Verification items for this drawing (mm, ordinates from the low corner). Coordinates: 2 decimals unless noted, no trailing zeros. Loops run counter-clockwise (first coordinate to the right, second up) from the corner with the lowest first, then second, coordinate; pieces in that order, holes last. Notation, with made-up numbers: (-35, 58) -> (24, 58) arc R13 ccw to (24, 75) -> close; hole circle Ø7 at (48, 17.25). An arc over 180 degrees is marked (long way). Write item = value, one per line.
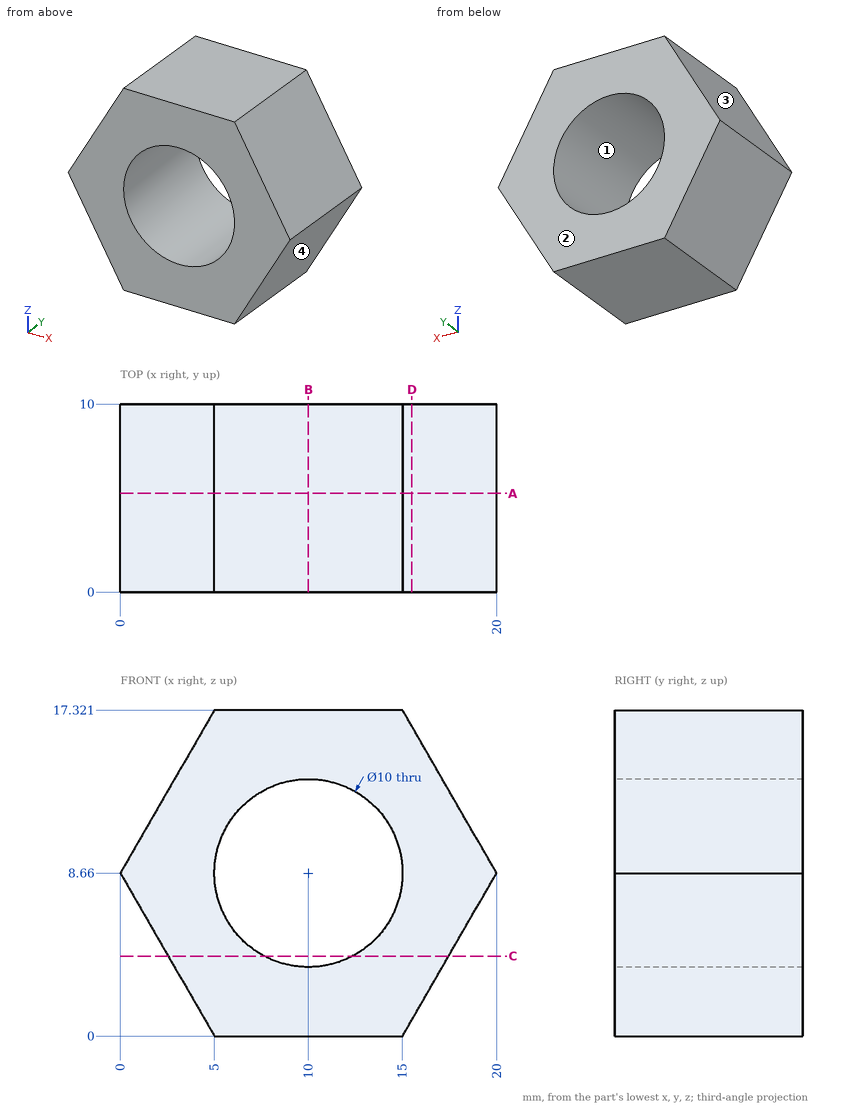
1) Sectioned sample at C-C, the plane z = 4.25. Record the cut outline in (x, y) (1 decimal), plus the area to 3 significant figures.
Ans:
outline = (2.5, 0) -> (7.6, 0) -> (7.6, 10) -> (2.5, 10) -> close; (12.4, 0) -> (17.5, 0) -> (17.5, 10) -> (12.4, 10) -> close
area = 102 mm2
2) Sectioned sample at B-B, the plane x = 10. Record the cut outline in (y, z).
Ans:
outline = (0, 0) -> (10, 0) -> (10, 3.66) -> (0, 3.66) -> close; (0, 13.66) -> (10, 13.66) -> (10, 17.32) -> (0, 17.32) -> close
3) Sectioned sample at A-A, the plane y = 5.25. Record the cut outline in (x, z).
Ans:
outline = (0, 8.66) -> (5, 0) -> (15, 0) -> (20, 8.66) -> (15, 17.32) -> (5, 17.32) -> close; hole circle Ø10 at (10, 8.66)
4) Release check for a two-part mould opening along Z. For the marked faces 1, 2, 3 and 4 record: pulls with the +Z half, pulls with the -Z half, needs draft (parallel to the pull), parting line crosses it, or undercut.
Ans:
face_1 = undercut
face_2 = needs draft
face_3 = pulls with the +Z half
face_4 = pulls with the -Z half
5) Sectioned sample at D-D, the plane x = 15.5. Record the cut outline in (y, z) (1 decimal).
Ans:
outline = (0, 0.9) -> (10, 0.9) -> (10, 16.5) -> (0, 16.5) -> close
6) Material ranges on line 1 (Z direction, x = 10, y = 6.5); line 2 (X direction, y = 8, z = 4.75) (1 decimal); line 3 (Z direction, x = 9.25, y = 5.5), recorded low to high.
Ans:
line_1 = 0 to 3.66, 13.66 to 17.32
line_2 = 2.3 to 6.9, 13.1 to 17.7
line_3 = 0 to 3.72, 13.6 to 17.32
